Geometry check sheet. Reference: the model listing, model coordinates, mm. A direction names the side the tool comes from. Coordinates: 2 decimals unless noted, no trailing zeros. Order: outer loops, then holes, each group sorted by start corner. A loop starts at its lowest first (then second) coordinate and runs counter-clockwise, first axis right, second up. Notation, with made-up numbers: (16, 9.5) - (46, 9.5) arc R28 cw to (46, 42.5) - close; hole circle Ø3 at (-22, 28). An arc over 180 degrees is marked (long way). Put each result on its own line as item: value.
from build123d import *

# Parameters (mm, degrees)
SKETCH2_R           = 125
BOSS_EXTRUDE1_DEPTH = 1000
SKETCH7_R           = 30
BOSS_EXTRUDE3_DEPTH = 145
BOSS_EXTRUDE4_START = 300
SKETCH8_R           = 30
BOSS_EXTRUDE4_DEPTH = 300
SKETCH9_W           = 18
SKETCH9_H           = 11
CUT_EXTRUDE1_DEPTH  = 60


with BuildPart() as part:
    # Sketch2 → Boss-Extrude1 (new body)
    with BuildSketch(Plane.XY):
        Circle(SKETCH2_R)
    extrude(amount=BOSS_EXTRUDE1_DEPTH)

    # Sketch7 → Boss-Extrude3 (add)
    with BuildSketch(Plane.XY.offset(1000)):
        Circle(SKETCH7_R)
    extrude(amount=BOSS_EXTRUDE3_DEPTH)

    # Sketch8 → Boss-Extrude4 (add)
    with BuildSketch(Plane(origin=(0, 0, 0), x_dir=(-1, 0, 0), z_dir=(0, 0, -1)).offset(BOSS_EXTRUDE4_START)):
        with Locations(Location((0, 0, 0), (0, 0, 180))):
            Circle(SKETCH8_R)
    extrude(amount=-BOSS_EXTRUDE4_DEPTH)

    # Sketch9 → Cut-Extrude1 (cut)
    with BuildSketch(Plane(origin=(0, 0, -300), x_dir=(-1, 0, 0), z_dir=(0, 0, -1))):
        with Locations((0, 30)):
            Rectangle(SKETCH9_W, SKETCH9_H)
    extrude(amount=-CUT_EXTRUDE1_DEPTH, mode=Mode.SUBTRACT)


solid = part.part
Q1. Depth check by flat-ended pin: pin 1 Ø3 at (x, z) = (-16.5, -72.5) entering from +Y; pin 2 Ø4 at (x, y) = (44.5, -31) entering from +Z; pin 3 Ø2 at (y, z) = (-80.5, 809) entering from +X. Enter the tip coordinate at first touch or a pass-through.
Answer block:
pin 1: stops at y = 25.98
pin 2: stops at z = 1000
pin 3: stops at x = 96.46
Q2. Thickness scan on L1, parallel to Z at x = 4.5, y = 44.5; L2, parallel to X at y = -3.5, z = -25.5; L3, parallel to X at y = -58, z = 838.5. Record the ranges inside material, lowest first. Write a range as [from, to].
Answer block:
L1: z = [0, 1000]
L2: x = [-29.8, 29.8]
L3: x = [-110.73, 110.73]
Q3. Section check D-D on z = 589.5. Record the boundary of the cut face in (x, y).
Answer block:
outline: circle Ø250 at (0, 0)
Q4. Access from +Z, -Z, +X, -X, +Y, -Y to the whole of each face (thin tool, end or side, straight path). Record for faces 1 (the flat face through (26, -26, 0)), 2 (the flat face through (26, -26, 1000)), 3 (the flat face through (0, 0, 1145)).
Answer block:
face 1: -Z
face 2: +Z
face 3: +Z, +X, -X, +Y, -Y
Q5. Section check B-B on z = -137.5. Record the boundary of the cut face in (x, y), then the cut area to 3 significant figures.
Answer block:
outline: circle Ø60 at (0, 0)
area: 2,830 mm^2
Q6. Section check C-C on x = -60.5. Record the boundary of the cut face in (y, z).
Answer block:
outline: (-109.38, 0) - (109.38, 0) - (109.38, 1000) - (-109.38, 1000) - close
Q7. Section check A-A on y = 0. Record the boundary of the cut face in (x, z).
Answer block:
outline: (-125, 0) - (-30, 0) - (-30, -300) - (30, -300) - (30, 0) - (125, 0) - (125, 1000) - (30, 1000) - (30, 1145) - (-30, 1145) - (-30, 1000) - (-125, 1000) - close
